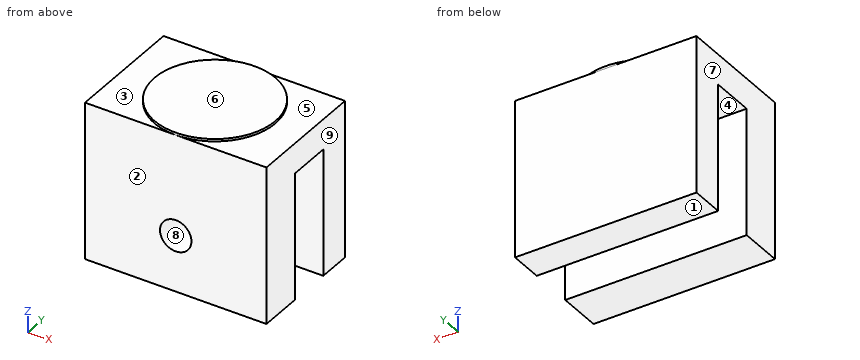
Autodesk Inventor part; units mm, degrees
ref_plane "YZ Plane" through (0, 0, 0) normal (1, 0, 0) x (0, 1, 0)
ref_plane "XZ Plane" through (0, 0, 0) normal (0, 1, 0) x (-1, 0, 0)
ref_plane "XY Plane" through (0, 0, 0) normal (0, 0, 1) x (1, 0, 0)
sketch "Sketch1" plane through (0, 0, 0) normal (1, 0, 0) x (0, 1, 0)
  line L0 (18.0976, -11.9743) -> (30.7976, -11.9743)
  line L1 (30.7976, -11.9743) -> (30.7976, -28.4843)
  line L2 (18.0976, -28.4843) -> (18.0976, -11.9743)
  line L3 (27.2855, -28.4843) -> (27.2855, -15.1493)
  line L4 (27.2855, -15.1493) -> (22.6756, -15.1493)
  line L5 (22.6756, -15.1493) -> (22.6756, -28.4843)
  line L6 (30.7976, -28.4843) -> (27.2855, -28.4843)
  line L7 (22.6756, -28.4843) -> (18.0976, -28.4843)
  point P0 (0, 0)
  dimension "d0" = 12.7
  dimension "d1" = 16.51
  dimension "d14" = 3.175
extrude "Extrusion1" add sketch "Sketch1" along normal blind 19.05
sketch "Sketch2" plane through (0, 18.0976, -28.4843) normal (0, -1, 0) x (1, 0, 0)
  circle A0 centre (9.525, 5.8867) radius 2.6491
  point P0 (0, 28.4843)
hole "Hole1" at (9.525, 18.0976, -22.5976) direction (0, 1, 0) diameter 3.302 depth 7.62 tip angle 118
sketch "Sketch3" plane through (0, 18.0976, -11.9743) normal (0, 0, 1) x (1, 0, 0)
  circle A0 centre (9.525, 6.35) radius 6.35
  point P0 (0, -18.0976)
  dimension "d11" = 12.7
extrude "Extrusion2" add sketch "Sketch3" along normal blind 0.254
properties part number "endcapTarget"
Geometry check sheet. Reference: the model listing, model coordinates, mm. Face numbers are marked on the shaded views. A direction names the side the tool comes from. Round coordinates to 2 decimals unless told otherwise and drop trailing zeros. Write each loop counter-clockwise with the first axis right and the second up, starting at its lowest first coordinate (ties: lowest second). Pieces come first, ordered by that corner, then holes. Notation, with made-up numbers: (83, 8) -> (133, 8) arc R29 cw to (133, 43) -> close; hole circle Ø9 at (87.5, 52). An arc over 180 degrees is marked (long way). One line per item, written item: value. Start each with the question number.
(1) Cross-section at D-D, the plane y = 26.25. Record the cut outline in (x, z), and give its area (3 significant figures).
(2) Draft check along X on the marked faces 6, 7, 8 and 9. Enter one of: +X half, -X half, draft (parallel to the pull), parting line (faces both ways), or undercut.
(3) Scan lines: line 1 (Y direction, x = 1.5, z = -15.25); line 2 (Z direction, x = 3, y = 25.25); line 3 (Z direction, x = 15, y = 19.75). Record each from-to range of solid material in increasing order. Write a range as [from, to].
(4) Cross-section at C-C, the plane z = -23. Record the cut outline in (x, y).
(5) Access from +Z, -Z, +X, -X, +Y, -Y to the whole of each face (thin tool, end or side, straight path). Record for the marked faces 1, 2, 3, 4 and 5.
(6) Cross-section at A-A, the plane z = -20.5. Record the cut outline in (x, y).
(7) Cross-section at B-B, the plane x = 10.5. Record the cut outline in (y, z).
(8) Go/stop test with a flat-tipped pin: pin 1 Ø3.5 at (x, y) = (11.5, 24.5) entering from -Z. Record where the tip stops, or that it passes through.
Answer:
1. outline: (0, -15.15) -> (19.05, -15.15) -> (19.05, -11.97) -> (15.61, -11.97) -> (15.61, -11.72) -> (3.44, -11.72) -> (3.44, -11.97) -> (0, -11.97) -> close
1. area: 63.6 mm²
2. face 6: draft
2. face 7: -X half
2. face 8: undercut
2. face 9: +X half
3. line 1: [18.1, 22.68], [27.29, 30.8]
3. line 2: [-15.15, -11.97]
3. line 3: [-28.48, -11.97]
4. outline: (0, 18.1) -> (7.92, 18.1) -> (7.92, 22.68) -> (0, 22.68) -> close; (0, 27.29) -> (19.05, 27.29) -> (19.05, 30.8) -> (0, 30.8) -> close; (11.13, 18.1) -> (19.05, 18.1) -> (19.05, 22.68) -> (11.13, 22.68) -> close
5. face 1: -Z, +X, -X, +Y, -Y
5. face 2: +Z, -Z, +X, -X, -Y
5. face 3: +Z, -X
5. face 4: -Z, +X, -X
5. face 5: +Z, +X
6. outline: (0, 18.1) -> (19.05, 18.1) -> (19.05, 22.68) -> (0, 22.68) -> close; (0, 27.29) -> (19.05, 27.29) -> (19.05, 30.8) -> (0, 30.8) -> close
7. outline: (18.1, -28.48) -> (22.68, -28.48) -> (22.68, -23.93) -> (18.1, -23.93) -> close; (18.1, -21.27) -> (22.68, -21.27) -> (22.68, -15.15) -> (27.29, -15.15) -> (27.29, -28.48) -> (30.8, -28.48) -> (30.8, -11.97) -> (30.72, -11.97) -> (30.72, -11.72) -> (18.17, -11.72) -> (18.17, -11.97) -> (18.1, -11.97) -> close
8. pin 1: z = -15.15
